from build123d import *

# Parameters (mm, degrees)
F1_R     = 100
F2_DEPTH = 400
F3_R     = 10
F4_DEPTH = 150
F5_R     = 10
F6_DEPTH = 150


with BuildPart() as f2:
    # F1 (on offset) → F2 (new body)
    with BuildSketch(Plane.XY.offset(200)):
        Circle(F1_R)
    extrude(amount=-F2_DEPTH)

    # F3 (on Front) → F4 (join)
    with BuildSketch(Plane.XZ):
        with Locations((-89, 189)):
            Circle(F3_R)
    extrude(amount=F4_DEPTH)

    # F5 (on Front) → F6 (join)
    with BuildSketch(Plane.XZ):
        with Locations((89, -189)):
            Circle(F5_R)
    extrude(amount=-F6_DEPTH)


solid = f2.part
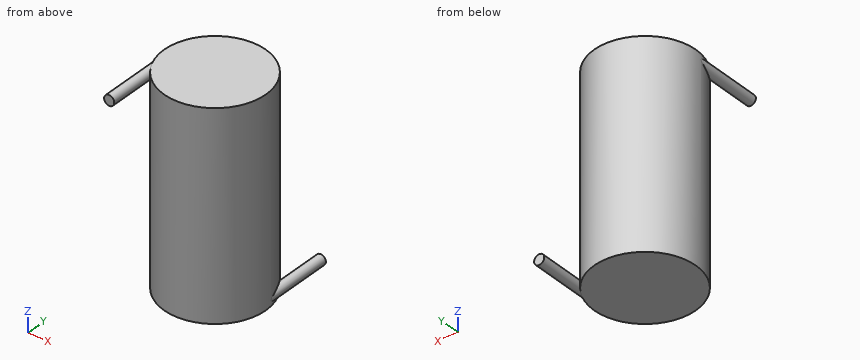
Input: part model. Units: mm. Frame: model coordinates. Give positions to 0.01 mm unless a question says otherwise; leave off trailing zeros. Loops run counter-clockwise (first coordinate to the right, second up) from the corner with the lowest first, then second, coordinate; pieces in that order, holes last. Notation, with made-up numbers: (34, -20.5) -> (92, -20.5) arc R30 cw to (92, 18.5) -> close; hole circle Ø2 at (-22, 46). An arc over 180 degrees is marked (long way). Answer as a JSON object with one key per item and string values. Group by question number.
Item 1: Cut plane A-A, the plane x = -89. Return the cut outline in (y, z), and give its area (3 significant figures).
Item 2: Pin query (flat end, axial travel): P1, Ø2, axis at y = 64.5, z = -149, coming from the -X side; P2, Ø3, axis at y = 16.5, z = -44.5, coming from the -X side; P3, Ø6, axis at x = -64.5, z = 160, coming from the -Y side. Return the tip coordinate at first contact, or that it passes through.
Item 3: Cut plane D-D, the plane x = 0. Return the cut outline in (y, z), and give its area (3 significant figures).
Item 4: Cut plane B-B, the plane z = -53. Return the cut outline in (x, y), and give its area (3 significant figures).
Item 5: Line query: probe 1 along Y at (x, z) = (-13.5, 25.5); probe 2 along Y at (x, z) = (61.5, 118.5); probe 3 along X at (y, z) = (34, 180). Output: solid intervals per line, ascending.
Item 6: Cut plane C-C, the plane y = -130. Return the cut outline in (x, z), and give its area (3 significant figures).
Checks:
{
 "1": {"outline": "(-150, 179) -> (-45.6, 179) -> (-45.6, -200) -> (45.6, -200) -> (45.6, 200) -> (-45.6, 200) -> (-45.6, 199) -> (-150, 199) -> close", "area": "38,600 mm²"},
 "2": {"P1": "stops at x = -77.25", "P2": "stops at x = -98.87", "P3": "stops at y = -78.85"},
 "3": {"outline": "(-100, -200) -> (100, -200) -> (100, 200) -> (-100, 200) -> close", "area": "80,000 mm²"},
 "4": {"outline": "circle Ø200 at (0, 0)", "area": "31,400 mm²"},
 "5": {"probe 1": "y = -99.08 to 99.08", "probe 2": "y = -78.85 to 78.85", "probe 3": "x = -94.04 to 94.04"},
 "6": {"outline": "circle Ø20 at (-89, 189)", "area": "314 mm²"}
}
